Could you check a few things on this drawing? It's one solid part, dimensions in mm from its lowest x, y, z. Give positions to 0.01 mm unless a question says otherwise; leave off trailing zeros. Order: outer loops, then holes, each group sorted by start corner. A loop starts at its lowest first (then second) coordinate and runs counter-clockwise, first axis right, second up.
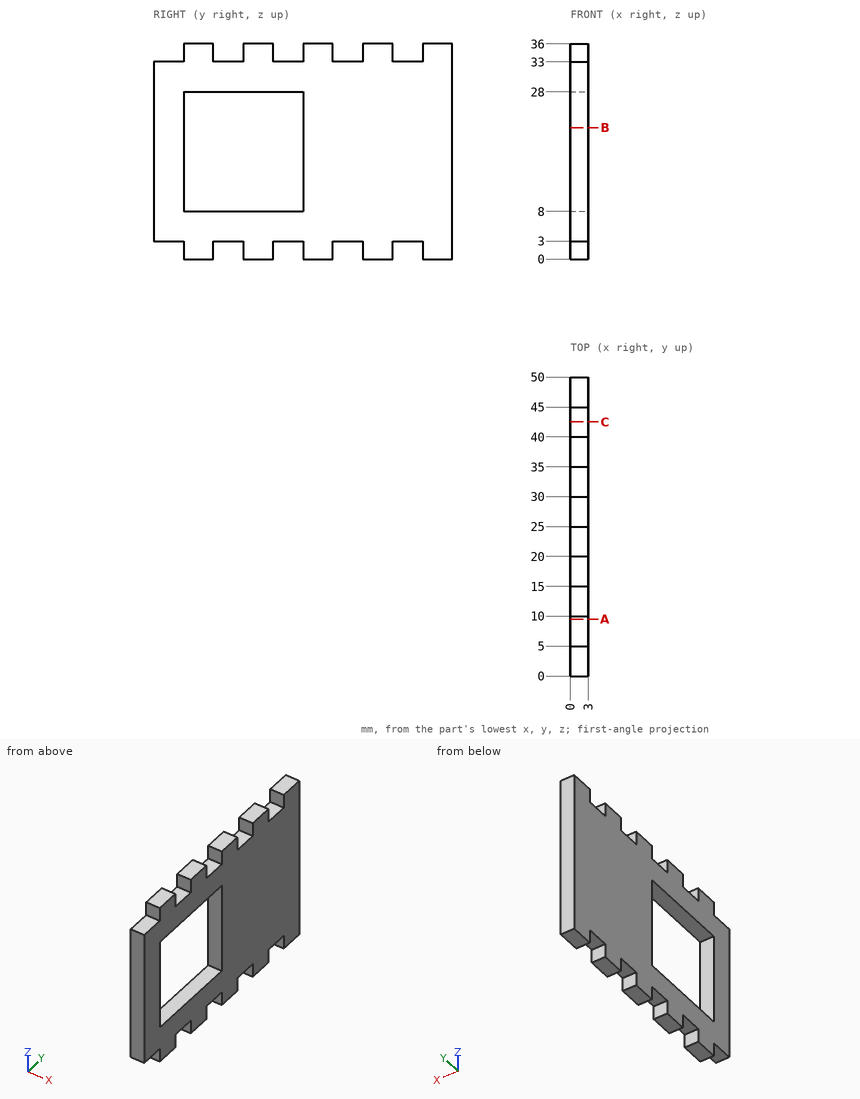
1) I'm going to push flat-ended pins straight in: pin 1 Ø1.5 at (x, z) = (2, 34.5) entering from -Y; pin 2 Ø0.9 at (x, y) = (1.5, 13.5) entering from -Z. Where does each tip first touch, or does it pass through?
2) Suppose I cut it at C-C (y = 42.5). Please give me the cut outline in (x, z), and give its area (3 significant figures).
3) Suppose I cut it at B-B (z = 22). Please give me the cut outline in (x, y), and give its area (3 significant figures).
4) If I drill on line 1 (Y direction, x = 0.45, z = 2.5); line 2 (Y direction, x = 0.7, z = 15); line 3 (Z direction, x = 0.2, y = 41), over which ranges is the centre line in solid material (lowest first)?
5) Suppose I cut it at A-A (y = 9.5). Please give me the cut outline in (x, z), and give its area (3 significant figures).
Results:
1. pin 1: stops at y = 5
1. pin 2: stops at z = 3
2. outline: (0, 3) - (3, 3) - (3, 33) - (0, 33) - close
2. area: 90.0 mm2
3. outline: (0, 0) - (3, 0) - (3, 5) - (0, 5) - close; (0, 25) - (3, 25) - (3, 50) - (0, 50) - close
3. area: 90.0 mm2
4. line 1: y = 5 to 10, 15 to 20, 25 to 30, 35 to 40, 45 to 50
4. line 2: y = 0 to 5, 25 to 50
4. line 3: z = 3 to 33
5. outline: (0, 0) - (3, 0) - (3, 8) - (0, 8) - close; (0, 28) - (3, 28) - (3, 36) - (0, 36) - close
5. area: 48.0 mm2
